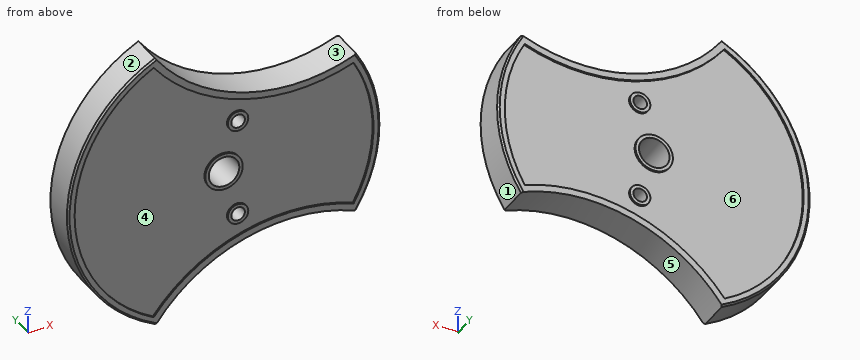
Autodesk Inventor part; units mm, degrees
ref_plane "YZ Plane" through (0, 0, 0) normal (1, 0, 0) x (0, 1, 0)
ref_plane "XZ Plane" through (0, 0, 0) normal (0, 1, 0) x (-1, 0, 0)
ref_plane "XY Plane" through (0, 0, 0) normal (0, 0, 1) x (1, 0, 0)
sketch "Sketch1" plane through (0, 0, 0) normal (0, 1, 0) x (-1, 0, 0)
  arc A0 (-38.9896, 24.4092) -> (-38.9896, -24.4092) centre (0, 0) ccw
  arc A1 (-38.9896, 24.4092) -> (20.1302, 41.3615) centre (-20.1215, 70.1721) ccw
  line L0 (0, 0) -> (-20.1215, 70.1721) construction
  line L1 (102.2, 0) -> (-102.2, 0) construction
  circle A2 centre (0, 0) radius 73 construction
  arc A3 (20.1302, -41.3615) -> (-38.9896, -24.4092) centre (-20.1215, -70.1721) ccw
  line L2 (20.1302, 41.3615) -> (20.1302, -41.3615) construction
  line L3 (-38.9896, 24.4092) -> (-38.9896, -24.4092) construction
  arc A4 (-12.6793, 44.218) -> (-38.9896, 24.4092) centre (0, 0) ccw construction
  arc A5 (20.1302, 41.3615) -> (-12.6793, 44.218) centre (0, 0) ccw construction
  arc A6 (20.1302, -41.3615) -> (20.1302, 41.3615) centre (0, 0) ccw
  arc A7 (-38.9896, -24.4092) -> (20.1302, -41.3615) centre (0, 0) ccw construction
  dimension "d3" = 146
  dimension "d0" = 92
  dimension "d1" = 49.5
  dimension "d2" = 74
extrude "Extrusion1" add sketch "Sketch1" along normal mid plane 10
sketch "Sketch6" plane through (0, 5, 0) normal (0, 1, 0) x (1, 0, 0)
  arc A0 (-20.1302, 41.3615) -> (-20.1302, -41.3615) centre (0, 0) ccw
  arc A1 (38.9896, -24.4092) -> (-20.1302, -41.3615) centre (20.1215, -70.1721) ccw
  arc A2 (38.9896, -24.4092) -> (38.9896, 24.4092) centre (0, 0) ccw
  arc A3 (-20.1302, 41.3615) -> (38.9896, 24.4092) centre (20.1215, 70.1721) ccw
  line L0 (0, 0) -> (20.1215, -70.1721) construction
  line L1 (0, 0) -> (20.1215, 70.1721) construction
  point P0 (4.1346, -14.4189)
  point P1 (4.1346, 14.4189)
  dimension "d15" = 15
hole "Hole1" at (4.1346, 5, 14.4189) at (4.1346, 5, -14.4189) direction (0, -1, 0) diameter 4 end through all
sketch "Sketch7" plane through (0, 5, 0) normal (0, 1, 0) x (1, 0, 0)
  circle A0 centre (4.1346, -14.4189) radius 2
  circle A1 centre (4.1346, 14.4189) radius 2
  arc A2 (-20.1302, 41.3615) -> (-20.1302, -41.3615) centre (0, 0) ccw
  arc A3 (38.9896, -24.4092) -> (-20.1302, -41.3615) centre (20.1215, -70.1721) ccw
  arc A4 (38.9896, -24.4092) -> (38.9896, 24.4092) centre (0, 0) ccw
  arc A5 (-20.1302, 41.3615) -> (38.9896, 24.4092) centre (20.1215, 70.1721) ccw
  arc A6 (-20.7288, 38.8113) -> (-20.7288, -38.8113) centre (0, 0) ccw
  arc A7 (-20.7288, 38.8113) -> (38.1459, 21.9293) centre (20.1215, 70.1721) ccw
  arc A8 (38.1459, -21.9293) -> (38.1459, 21.9293) centre (0, 0) ccw
  arc A9 (38.1459, -21.9293) -> (-20.7288, -38.8113) centre (20.1215, -70.1721) ccw
  circle A10 centre (4.1346, -14.4189) radius 3
  circle A11 centre (4.1346, 14.4189) radius 3
  circle A12 centre (0, 0) radius 5.5
  dimension "d23" = 2
  dimension "d24" = 6
  dimension "d25" = 6
  dimension "d35" = 11
extrude "Extrusion3" cut sketch "Sketch7" against normal blind 0.5 contours A7 A8 A9 A6
hole "Hole2" at (0, 5, 0) direction (0, -1, 0) diameter 9 end through all
chamfer "Chamfer2" distance 0.5 angle 45 2 edges at (-46, 5, 0) (46, 5, 0)
mirror "Mirror2" about plane through (0, 0, 0) normal (0, 1, 0) of "Extrusion3"
chamfer "Chamfer3" distance 0.5 angle 45 2 edges at (46, -5, 0) (-46, -5, 0)
properties part number "Disk"
Could you check a few things on this model? Use its own coordinates, in mm. Face numbers are marked on the shaded views. A direction names the side the tool comes from. Round coordinates to 2 decimals unless told otherwise and drop trailing zeros. Write each loop counter-clockwise with the first axis right and the second up, starting at its lowest first coordinate (ties: lowest second). Pieces come first, ordered by that corner, then holes.
(1) For pin 1 (4.5 mm diameter, centred on x = 4.13, z = 14.42, fed in from -Y); pin 2 (5.5 mm diameter, centred on x = 0, z = 0, fed in from +Y); pin 3 (10 mm diameter, centred on x = -21, z = -15.5, fed in from +Y); pin 4 (1 mm diameter, centred on x = -24, y = 1.5, fed in from +Z), each with a flat end and sliding along its axis, tell me the tip position at first contact or that it passes through.
Findings below:
pin 1: stops at y = -5
pin 2: passes through
pin 3: stops at y = 4.5
pin 4: stops at z = 39.54
(2) Suppose I cut it at B-B on y = 3. Write out the boundary of the cut face in (x, z), and give its area (3 significant figures).
Findings below:
outline: (-20.13, -41.36) arc R49.5 cw to (38.99, -24.41) arc R46 ccw to (38.99, 24.41) arc R49.5 cw to (-20.13, 41.36) arc R46 ccw to start; hole circle Ø9 at (0, 0); hole circle Ø4 at (4.13, -14.42); hole circle Ø4 at (4.13, 14.42)
area: 4,660 mm2
(3) Thinking about a two-plate mould opening in X: for the marked faces 1, 2 and 3, which applies, +X half, -X half, draft (parallel to the pull), parting line (faces both ways), or undercut?
Findings below:
face 1: +X half
face 2: -X half
face 3: undercut
(4) If I drill on probe 1 along X at (y, z) = (1.75, 0); probe 2 along Y at (x, z) = (-23.5, 26.5); probe 3 along Z at (x, y) = (4, -4), over which ranges is the centre line in solid material (lowest first)?
Findings below:
probe 1: x = -46 to -4.5, 4.5 to 46
probe 2: y = -4.5 to 4.5
probe 3: z = -23.37 to -16.41, -12.42 to -2.06, 2.06 to 12.42, 16.41 to 23.37
(5) Which directions (+Z, -Z, +X, -X, +Y, -Y) give clear straight access to the entire face, cutting with the end or side of a thin tool? Please do the marked faces 4, 5 and 6.
Findings below:
face 4: -Y
face 5: -Z, +Y, -Y
face 6: +Y
(6) Suppose I cut it at A-A on z = 0. Write out the boundary of the cut face in (x, y), and give its area (4 significant figures).
Findings below:
outline: (-46, -4.5) - (-45.5, -5) - (-44, -5) - (-44, -4.5) - (-5.5, -4.5) - (-5.5, -5) - (-4.5, -5) - (-4.5, 5) - (-5.5, 5) - (-5.5, 4.5) - (-44, 4.5) - (-44, 5) - (-45.5, 5) - (-46, 4.5) - close; (4.5, -5) - (5.5, -5) - (5.5, -4.5) - (44, -4.5) - (44, -5) - (45.5, -5) - (46, -4.5) - (46, 4.5) - (45.5, 5) - (44, 5) - (44, 4.5) - (5.5, 4.5) - (5.5, 5) - (4.5, 5) - close
area: 752.5 mm2
